from build123d import *

# Parameters (mm, degrees)
SKETCH_1_R           = 1
EXTRUDE_1_DEPTH      = 24
SKETCH_2_W           = 8
SKETCH_2_H           = 4
CUT_EXTRUDE_2_DEPTH  = 4
CUT_EXTRUDE_3_DEPTH  = 6
CUT_EXTRUDE_START    = -7
CUT_EXTRUDE_4_DEPTH  = 12
SKETCH_4_W           = 2
SKETCH_4_H           = 1
EXTRUDE_2_DEPTH      = 0.5
CUT_EXTRUDE_21_DEPTH = 0.5
CUT_EXTRUDE_22_DEPTH = 0.5


with BuildPart() as part:
    # 草图1 → 凸台-拉伸1 (new body)
    with BuildSketch(Plane.XY):
        with BuildLine():
            Line((0, 2), (47, 2))
            Line((47, 2), (47, -6))
            Line((47, -6), (45, -6))
            Line((45, -6), (45, -2))
            Line((45, -2), (0, -2))
            ThreePointArc((0, -2), (-2, 0), (0, 2))
        make_face()
        Circle(SKETCH_1_R, mode=Mode.SUBTRACT)
    extrude(amount=EXTRUDE_1_DEPTH)

    # 草图2 → 切除-拉伸2 (cut)
    with BuildSketch(Plane.XY.offset(24)):
        Rectangle(SKETCH_2_W, SKETCH_2_H)
    extrude(amount=-CUT_EXTRUDE_2_DEPTH, mode=Mode.SUBTRACT)

    # 草图3 → 切除-拉伸3 (cut)
    with BuildSketch(Plane(origin=(0, 0, 0), x_dir=(-1, 0, 0), z_dir=(0, 0, -1))):
        with BuildLine():
            Line((0, 2), (-4, 2))
            Line((-4, 2), (-4, -2))
            Line((-4, -2), (0, -2))
            ThreePointArc((0, -2), (2, 0), (0, 2))
        make_face()
    extrude(amount=-CUT_EXTRUDE_3_DEPTH, mode=Mode.SUBTRACT)

    # 草图3<2> → 切除-拉伸4 (cut)
    with BuildSketch(Plane(origin=(0, 0, 0), x_dir=(-1, 0, 0), z_dir=(0, 0, -1)).offset(CUT_EXTRUDE_START)):
        with BuildLine():
            ThreePointArc((0, -2), (2, 0), (0, 2))
            Line((0, 2), (-4, 2))
            Line((-4, 2), (-4, -2))
            Line((-4, -2), (0, -2))
        make_face()
    extrude(amount=-CUT_EXTRUDE_4_DEPTH, mode=Mode.SUBTRACT)

    # 草图4 → 凸台-拉伸2 (add)
    with BuildSketch(Plane.ZY.offset(-45)):
        with Locations((12, -5.5)):
            Rectangle(SKETCH_4_W, SKETCH_4_H)
    extrude(amount=EXTRUDE_2_DEPTH)

    # 草图5 → 切除-拉伸21 (cut)
    with BuildSketch(Plane.XY):
        Polygon((4, 2), (4, -2), (45, -2), (45, -6), (47, -6), (47, 2), align=None)
    extrude(amount=CUT_EXTRUDE_21_DEPTH, mode=Mode.SUBTRACT)

    # 草图6 → 切除-拉伸22 (cut)
    with BuildSketch(Plane.XY.offset(24)):
        Polygon((4, -2), (45, -2), (45, -6), (47, -6), (47, 2), (4, 2), align=None)
    extrude(amount=-CUT_EXTRUDE_22_DEPTH, mode=Mode.SUBTRACT)


solid = part.part
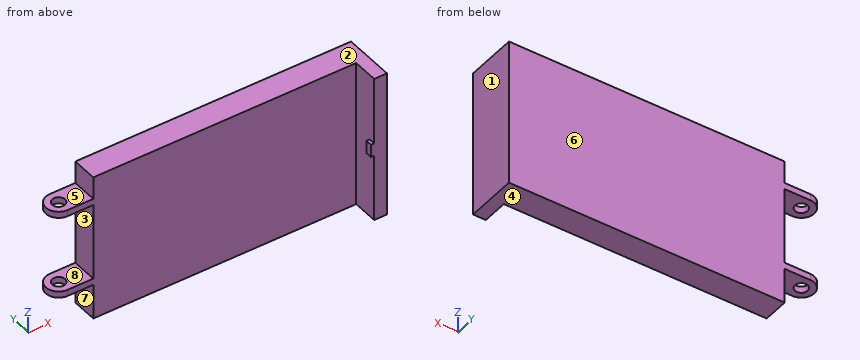
Design review of the part built by this model. Coordinates are the model's own, in mm. Face numbers are marked on the shaded views. A direction names the side the tool comes from. Give positions to 0.01 mm unless a question says otherwise; leave off trailing zeros. Loops run counter-clockwise (first coordinate to the right, second up) from the corner with the lowest first, then second, coordinate; pieces in that order, holes last. Notation, with made-up numbers: M 37.5,64 L 67.5,64 A29 cw 67.5,103 Z; hole C 67.5,-4 d1. An arc over 180 degrees is marked long. Answer as a JSON object with one key per item and string values.
Item 1: We need section C-C (x = 9.5). State the section outline as (y, z) points, and give its area (3 significant figures).
Output values:
{"outline": "M -2,0.5 L 2,0.5 L 2,23.5 L -2,23.5 Z", "area": "92.0 mm2"}
Item 2: We need section A-A (y = 0). State the section outline as (x, z) points.
Output values:
{"outline": "M -2,6 L -1,6 L -1,7 L -2,7 Z; M -2,19 L -1,19 L -1,20 L -2,20 Z; M 1,6 L 4,6 L 4,0.5 L 47,0.5 L 47,23.5 L 4,23.5 L 4,20 L 1,20 L 1,19 L 4,19 L 4,7 L 1,7 Z"}
Item 3: We need section B-B (z = 11.5). State the section outline as (x, y) points, and give its area (4 significant figures).
Output values:
{"outline": "M 4,-2 L 45,-2 L 45,-5 L 44.5,-5 L 44.5,-6 L 47,-6 L 47,2 L 4,2 Z", "area": "180.5 mm2"}
Item 4: We need section D-D (y = -3). State the section outline as (x, z) points.
Output values:
{"outline": "M 45,0.5 L 47,0.5 L 47,23.5 L 45,23.5 Z"}
Item 5: For P1, Ø1.6, axis at x = 0, y = 0, coming from the -Z side; P2, Ø3, axis at y = -4.5, z = 12, coming from the -X side; P3, Ø4.5, axis at y = 0.5, z = 15.5, coming from the -X side; P4, Ø12, axis at x = 20.5, z = 4, coming from the -Y side, all flat-tipped, find the tip position at first contact; note any pin that passes through.
Output values:
{"P1": "passes through", "P2": "stops at x = 44.5", "P3": "stops at x = 4", "P4": "stops at y = -2"}
Item 6: Wall thickness on line 1 along Y through (x, z) = (0, 6.6); line 2 along X through (y, z) = (0, 6.55); line 3 along Y through (x, z) = (44, 8.5): over which ranges is each line inside the solid? List them lowest first.
Output values:
{"line 1": "y = -2 to -1, 1 to 2", "line 2": "x = -2 to -1, 1 to 47", "line 3": "y = -2 to 2"}
Item 7: Machinability: for the marked faces 5, 6, 7 and 8, which of the approach directions +Z, -Z, +X, -X, +Y, -Y give a long, thin tool a straight path to every point of the face, cutting with its end or side? Answer none if there is none.
Output values:
{"face 5": "+Z, -X, +Y, -Y", "face 6": "+Z, -Z, +X, -X, +Y", "face 7": "-Z, -X, +Y, -Y", "face 8": "-X, +Y, -Y"}
Item 8: Mouldability with a two-part tool opening along Z and no side actions: class the marked faces 1, 2, 3 and 4 as pulls with the +Z half, pulls with the -Z half, needs draft (parallel to the pull), parting line crosses it, or undercut.
Output values:
{"face 1": "needs draft", "face 2": "pulls with the +Z half", "face 3": "undercut", "face 4": "pulls with the -Z half"}
